The model under review builds one solid part; all positions refer to its coordinate system, in mm. Face numbers are marked on the shaded views. A direction names the side the tool comes from. Give positions to 0.01 mm unless a question says otherwise; leave off trailing zeros. Loops run counter-clockwise (first coordinate to the right, second up) from the corner with the lowest first, then second, coordinate; pieces in that order, holes last. Notation, with made-up numbers: M 53.25,42.25 L 106.25,42.25 A23 cw 106.25,81.25 Z; hole C 36.25,53.5 d11. An arc over 180 degrees is marked long. Return JSON: item names as keys, results as strings. Group by question number.
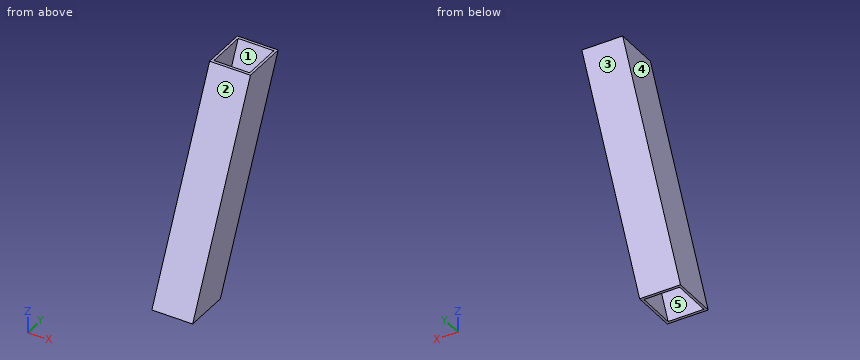
```python
from build123d import *

# Parameters (mm, degrees)
F1_DEPTH = 50.8
F2_T     = -3.175


with BuildPart() as f1:
    # F0 (on Right) → F1 (new body)
    with BuildSketch(Plane.YZ):
        Polygon((0, -36.428121), (117.0012, 214.481761), (60.949601, 214.481761), (-56.051598, -36.428121), align=None)
    extrude(amount=F1_DEPTH)

    # F2
    f2_openings = [f1.faces().sort_by_distance(p)[0] for p in [
        (25.4, -28.025799, -36.428121),
        (25.4, 88.975401, 214.481761),
    ]]
    offset(amount=F2_T, openings=f2_openings)


solid = f1.part
```
(1) For pin 1 (12 mm diameter, centred on x = 22.5, z = 58.5, fed in from -Y); pin 2 (6 mm diameter, centred on x = 28, y = 4.5, fed in from +Z); pin 3 (3 mm diameter, centred on x = 10, z = -4, fed in from +Y), all flat-tipped, find the tip position at first contact; note any pin that passes through.
(2) Add section D-D (y = 45). Write out the cut boundary in (x, z) (3 decimals).
(3) Add section B-B (z = 142). Write out the cut boundary in (x, y) (3 decimals).
(4) Add section C-C (y = 87). Write out the cut boundary in (x, z) (3 decimals), and give its area (3 significant figures).
(5) Add section A-A (x = 38). Write out the cut boundary in (y, z).
(6) For probe 1 along X at (y, z) = (53, 120) (3 decimals); probe 2 along Y at (x, z) = (20, 130); probe 3 along Y at (x, z) = (47.5, 43), list the stretches that pass through material, from the lowest coordinate up.
(7) Mouldability with a two-part tool opening along Y and no side actions: class the marked faces 3, 4 and 5 as released by +Y, released by -Y, zero draft, split by the parting line, or undercut.
(8) For the marked faces 1 and 2, list the 3-axis set-ups (+Z, -Z, +X, -X, +Y, -Y) from which the entire face can be reached by the end or side of a thin tool; tool diameter is ignored.
Verdict:
{
 "1": {"pin 1": "stops at y = -14.58", "pin 2": "stops at z = 99.86", "pin 3": "stops at y = 15.82"},
 "2": {"outline": "M 0,60.075 L 50.8,60.075 L 50.8,180.278 L 0,180.278 Z; hole M 3.175,67.587 L 47.625,67.587 L 47.625,172.765 L 3.175,172.765 Z"},
 "3": {"outline": "M 0,27.151 L 50.8,27.151 L 50.8,83.202 L 0,83.202 Z; hole M 3.175,30.654 L 47.625,30.654 L 47.625,79.699 L 3.175,79.699 Z"},
 "4": {"outline": "M 0,150.144 L 50.8,150.144 L 50.8,214.482 L 47.625,214.482 L 47.625,157.657 L 3.175,157.657 L 3.175,214.482 L 0,214.482 Z", "area": "742 mm²"},
 "5": {"outline": "M -56.05,-36.43 L -52.55,-36.43 L 64.45,214.48 L 60.95,214.48 Z; M -3.5,-36.43 L 0,-36.43 L 117,214.48 L 113.5,214.48 Z"},
 "6": {"probe 1": "x = 0 to 3.175, 47.625 to 50.8", "probe 2": "y = 21.56 to 25.06, 74.1 to 77.61", "probe 3": "y = -19.01 to -15.51, 33.53 to 37.04"},
 "7": {"face 3": "released by +Y", "face 4": "zero draft", "face 5": "undercut"},
 "8": {"face 1": "none", "face 2": "+Z, +X, -X, -Y"}
}
